Could you check a few things on this drawing? It's one solid part, dimensions in mm from its lowest x, y, z. Give positions to 0.01 mm unless a question says otherwise; leave off trailing zeros. Loops run counter-clockwise (first coordinate to the right, second up) from the corner with the lowest first, then second, coordinate; pieces in that order, holes last. Notation, with made-up numbers: M 82,26.5 L 113,26.5 A18 ccw 113,45.5 Z; hole C 50,10.5 d7. An arc over 180 degrees is marked long. Answer as CSV lines item,"result". Start each with the question number.
Item 1: If we mould it in two halves opening along Y, with no side actions, what happens to the marked faces 1, 2, 3 and 4? For each: released by +Y, released by -Y, zero draft, split by the parting line, or undercut.
Item 2: I want a section at D-D on z = 21. List the corners of the cut face in (x, y) for me.
Item 3: I want a section at C-C on y = 7.2. List the corners of the cut face in (x, z) for me, plus the area to 3 significant figures.
Item 4: I want a section at B-B on z = 28.5. List the corners of the cut face in (x, y) for me, plus the area to 3 significant figures.
Item 5: Will these pins go through, and if not, where does the flat tip stop? P1, Ø3, axis at x = 11, z = 3.5, coming from the -Y side; P2, Ø3, axis at x = 5, z = 26.5, coming from the +Y side; P3, Ø8, axis at x = 2, z = 19.5, coming from the -Y side.
Item 6: If I drill on line 1 along Y through (x, z) = (7.2, 30); line 2 along X through (y, z) = (8, 19) (1 decimal); line 3 along Z through (x, y) = (4.75, 8.25) (1 decimal), over which ranges is the centre line in solid material (lowest first)? Write a range as from..to.
Item 7: I want a section at A-A on x = 7.2. List the corners of the cut face in (y, z) for me.
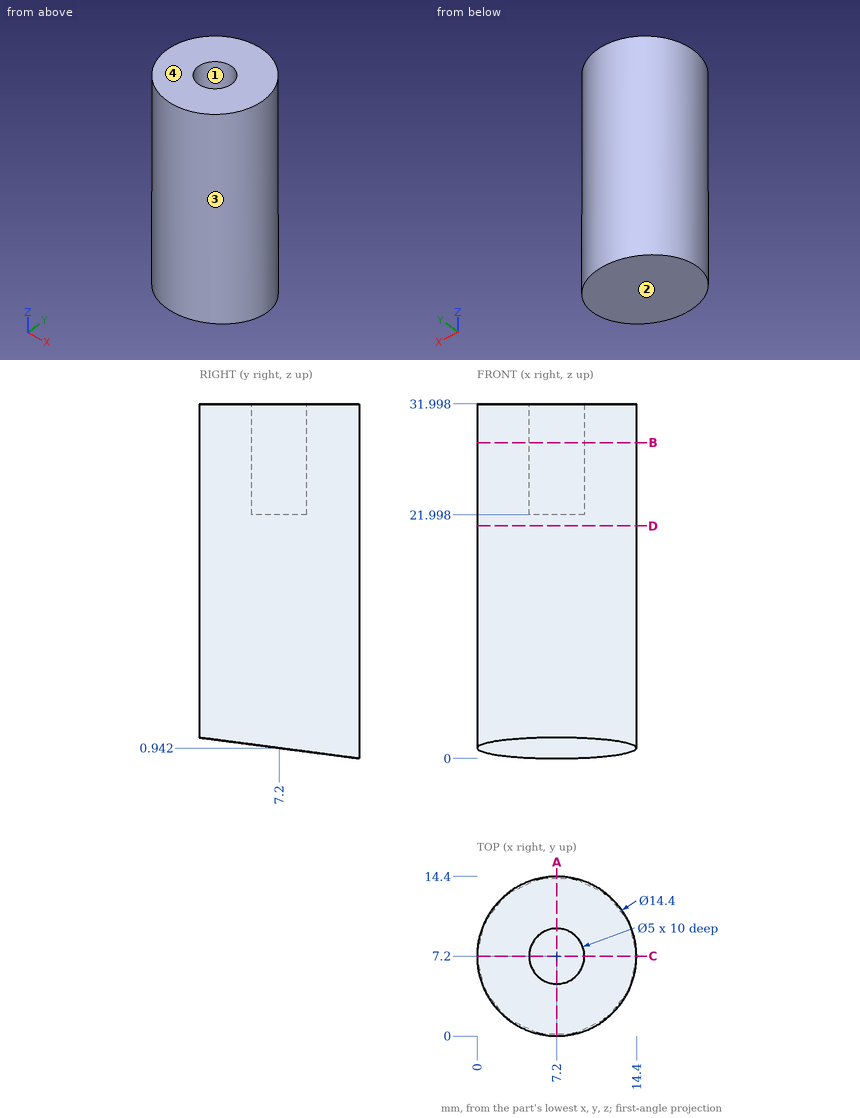
Result:
1,face 1,"undercut"
1,face 2,"released by -Y"
1,face 3,"split by the parting line"
1,face 4,"zero draft"
2,outline,"C 7.2,7.2 d14.4"
3,outline,"M 0,0.94 L 14.4,0.94 L 14.4,32 L 9.7,32 L 9.7,22 L 4.7,22 L 4.7,32 L 0,32 Z"
3,area,"397 mm^2"
4,outline,"C 7.2,7.2 d14.4; hole C 7.2,7.2 d5"
4,area,"143 mm^2"
5,P1,"y = 0.38"
5,P2,"y = 14.37"
5,P3,"y = 0.1"
6,line 1,"0..4.7, 9.7..14.4"
6,line 2,"0..14.4"
6,line 3,"0.8..32"
7,outline,"M 0,1.88 L 14.4,0 L 14.4,32 L 9.7,32 L 9.7,22 L 4.7,22 L 4.7,32 L 0,32 Z"
